Part print with two shaded views. Sizes in mm from the minimum x, y, z corner. Round coordinates to 2 decimals unless told otherwise and drop trailing zeros. Write each loop counter-clockwise with the first axis right and the second up, starting at its lowest first coordinate (ties: lowest second). Pieces come first, ordered by that corner, then holes. Notation, with made-up numbers: (6.25, -11.5) -> (30.25, -11.5) arc R29 ccw to (30.25, 26.5) -> close; hole circle Ø5 at (34.5, 89). An arc over 180 degrees is marked (long way). Put each result on its own line as item: value. Start each with the question number.
1. Saw through at D-D on x = 30. List the corners of the cut face in (y, z).
2. Drill centre lines: line 1 (X direction, y = 170, z = 1.3); line 2 (Y direction, x = 130, z = 3.55); line 3 (X direction, y = 100, z = 1.4). Where is each one in solid material? Low to high. Write a range as from..to.
3. Saw through at B-B on x = 210. List the corners of the cut face in (y, z).
4. Saw through at C-C on z = 1.85. State how many separate pieces and enclosed holes the cut face has, and give its area (3 significant figures).
5. Flat gauge pins, fed straight in: P1, Ø20.5, axis at x = 130, y = 30, coming from the +Z side; P2, Ø1.5, axis at y = 31, z = 0.5, coming from the -X side. Where does each tip first touch, or does it go through?
6. Saw through at A-A on y = 30. List the corners of the cut face in (x, z).
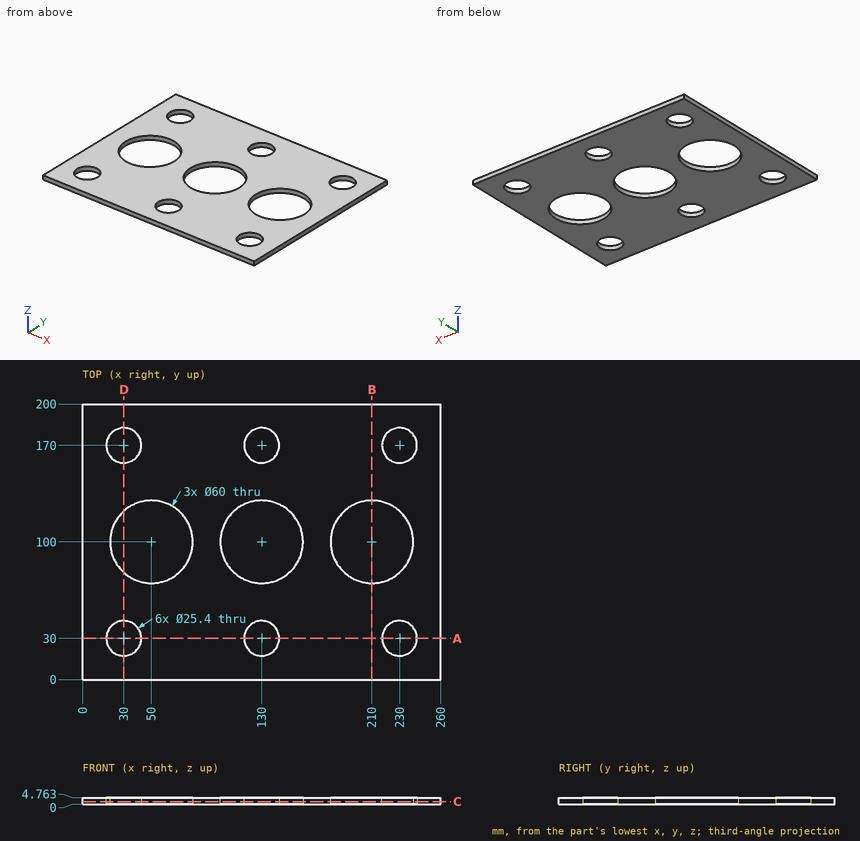
Return value:
1. outline: (0, 0) -> (17.3, 0) -> (17.3, 4.76) -> (0, 4.76) -> close; (42.7, 0) -> (77.64, 0) -> (77.64, 4.76) -> (42.7, 4.76) -> close; (122.36, 0) -> (157.3, 0) -> (157.3, 4.76) -> (122.36, 4.76) -> close; (182.7, 0) -> (200, 0) -> (200, 4.76) -> (182.7, 4.76) -> close
2. line 1: x = 0..17.3, 42.7..117.3, 142.7..217.3, 242.7..260
2. line 2: y = 0..17.3, 42.7..70, 130..157.3, 182.7..200
2. line 3: x = 0..20, 80..100, 160..180, 240..260
3. outline: (0, 0) -> (70, 0) -> (70, 4.76) -> (0, 4.76) -> close; (130, 0) -> (200, 0) -> (200, 4.76) -> (130, 4.76) -> close
4. separate pieces: 1
4. enclosed holes: 9
4. area: 40,500 mm^2
5. P1: passes through
5. P2: stops at x = 0
6. outline: (0, 0) -> (17.3, 0) -> (17.3, 4.76) -> (0, 4.76) -> close; (42.7, 0) -> (117.3, 0) -> (117.3, 4.76) -> (42.7, 4.76) -> close; (142.7, 0) -> (217.3, 0) -> (217.3, 4.76) -> (142.7, 4.76) -> close; (242.7, 0) -> (260, 0) -> (260, 4.76) -> (242.7, 4.76) -> close
